Build history of the part. All positions in model axes, mm. A direction names the side the tool comes from. Round coordinates to 2 decimals unless told otherwise and drop trailing zeros. Write each loop counter-clockwise with the first axis right and the second up, starting at its lowest first coordinate (ties: lowest second). Pieces come first, ordered by that corner, then holes. Notation, with made-up numbers: (-23, 47.25) -> (27, 47.25) arc R33 ccw to (27, 82.25) -> close; hole circle Ø11 at (39.25, 10.5). An arc over 180 degrees is marked (long way). Answer in a Markdown table with one row per item. Add a question column.
Autodesk Inventor part; units mm, degrees
ref_plane "YZ Plane" through (0, 0, 0) normal (1, 0, 0) x (0, 1, 0)
ref_plane "XZ Plane" through (0, 0, 0) normal (0, 1, 0) x (-1, 0, 0)
ref_plane "XY Plane" through (0, 0, 0) normal (0, 0, 1) x (1, 0, 0)
sketch "Szkic1" plane through (0, 0, 0) normal (0, 0, 1) x (1, 0, 0)
  circle A0 centre (0, 0) radius 12.5
  dimension "d0" = 25
extrude "Wyciągnięcie proste1" add sketch "Szkic1" along normal blind 32
sketch "Szkic2" plane through (0, 0, 32) normal (0, 0, 1) x (1, 0, 0)
  circle A0 centre (0, 0) radius 6
  dimension "d3" = 12
extrude "Wyciągnięcie proste2" cut sketch "Szkic2" against normal blind 32
sketch "Szkic3" plane through (0, 0, 0) normal (0, 1, 0) x (-1, 0, 0)
  circle A0 centre (-9, 5) radius 2
  circle A1 centre (-9, 27) radius 2
  line L0 (0, 0) -> (0, -10.8071)
  circle A2 centre (-9, 27) radius 3.5
  circle A3 centre (-9, 5) radius 3.5
  line L1 (-12.5, 0) -> (12.5, 0)
  line L2 (12.5, 32) -> (-12.5, 32)
  dimension "d6" = 4
  dimension "d7" = 4
  dimension "d8" = 9
  dimension "d9" = 9
  dimension "d10" = 7
  dimension "d11" = 7
  dimension "d12" = 5
  dimension "d13" = 5
extrude "Wyciągnięcie proste3" cut sketch "Szkic3" along normal blind 32 contours A0 | A1 | A2 | A3
sketch "Szkic4" plane through (0, 0, 0) normal (0, 1, 0) x (1, 0, 0)
  circle A0 centre (9, -27) radius 2.25
  circle A1 centre (9, -5) radius 2.25
  arc A2 (6, -6.8028) -> (12.5, -5) centre (9, -5) ccw
  arc A3 (12.5, -27) -> (6, -25.1972) centre (9, -27) ccw
  point P0 (0, 0)
  dimension "d16" = 4.5
  dimension "d17" = 4.5
extrude "Wyciągnięcie proste4" cut sketch "Szkic4" against normal blind 32
properties part number "Cartesian1_12_12_Clutch" material "Stal, stopowa"
(1) Saw through at B-B (z = 13.5). List the corners of the cut face in (x, y).
(2) Probe line 1 along Z through (x, y) = (9, -5.5); line 2 along X through (y, z) = (-3, 27); line 3 along X through (y, z) = (-5.5, 7). List the from-to ranges inside material, lowest first.
(3) Saw through at C-C (x = 10.5). List the corners of the cut face in (y, z).
(4) Saw through at A-A (x = 0). List the corners of the cut face in (y, z), plus the area to 3 significant figures.
(5) Drop flat-ended pins along their axis: P1, Ø6, axis at x = 9, z = 27, coming from the +Y side; P2, Ø4, axis at y = -5, z = 8.5, coming from the +X side; P3, Ø7, axis at x = 10, z = 5.5, coming from the +Y side. Give the stop position or say it passes through.
(6) Which spindle directions (+Z, -Z, +X, -X, +Y, -Y) get a long thin tool onto all of the face, cutting with end or side? Do faces 1 (the face through (-4.76, -3.65, 16.22)), 2 (the face through (11, 0, 3)). Say none if no direction does.
(7) Saw through at D-D (z = 26.5). List the corners of the cut face in (x, y), plus the area to 3 significant figures.
(8) Mould opens along Z. For faces 3 (the face through (11, 0, 25)), 4 (the face through (-3, -5.4, 32)), 5 (the face through (-3, -5.4, 0)) say: pulls with the +Z half, pulls with the -Z half, needs draft (parallel to the pull), parting line crosses it, or undercut.
Answer sheet:
| question | item | result |
|---|---|---|
| 1 | outline | circle Ø25 at (0, 0); hole circle Ø12 at (0, 0) |
| 2 | line 1 | z = 0 to 2.75, 7.25 to 24.75, 29.25 to 32 |
| 2 | line 2 | x = -12.13 to -5.2, 5.2 to 6.75, 11.25 to 12.13 |
| 2 | line 3 | x = -11.22 to -2.4, 2.4 to 7.97, 10.03 to 11.22 |
| 3 | outline | (-6.78, 0) -> (6.78, 0) -> (6.78, 1.84) -> (0, 1.84) -> (0, 3.32) -> (-6.78, 3.32) -> close; (-6.78, 6.68) -> (0, 6.68) -> (0, 8.16) -> (6.78, 8.16) -> (6.78, 23.84) -> (0, 23.84) -> (0, 25.32) -> (-6.78, 25.32) -> close; (-6.78, 28.68) -> (0, 28.68) -> (0, 30.16) -> (6.78, 30.16) -> (6.78, 32) -> (-6.78, 32) -> close |
| 4 | outline | (-12.5, 0) -> (-6, 0) -> (-6, 32) -> (-12.5, 32) -> close; (6, 0) -> (12.5, 0) -> (12.5, 32) -> (6, 32) -> close |
| 4 | area | 416 mm² |
| 5 | P1 | stops at y = 0 |
| 5 | P2 | stops at x = 12.13 |
| 5 | P3 | stops at y = 9.64 |
| 6 | face 1 | +Z, -Z |
| 6 | face 2 | +Y |
| 7 | outline | (5.54, 2.31) -> (5.54, 11.21) arc R12.5 ccw (long way) to (6.81, -10.48) -> (6.81, 0) -> (6, 0) arc R6 cw (long way) to start; (11.19, -5.56) arc R12.5 ccw to (12.46, 0.95) -> (12.46, 0) -> (11.19, 0) -> close |
| 7 | area | 286 mm² |
| 8 | face 3 | undercut |
| 8 | face 4 | pulls with the +Z half |
| 8 | face 5 | pulls with the -Z half |
